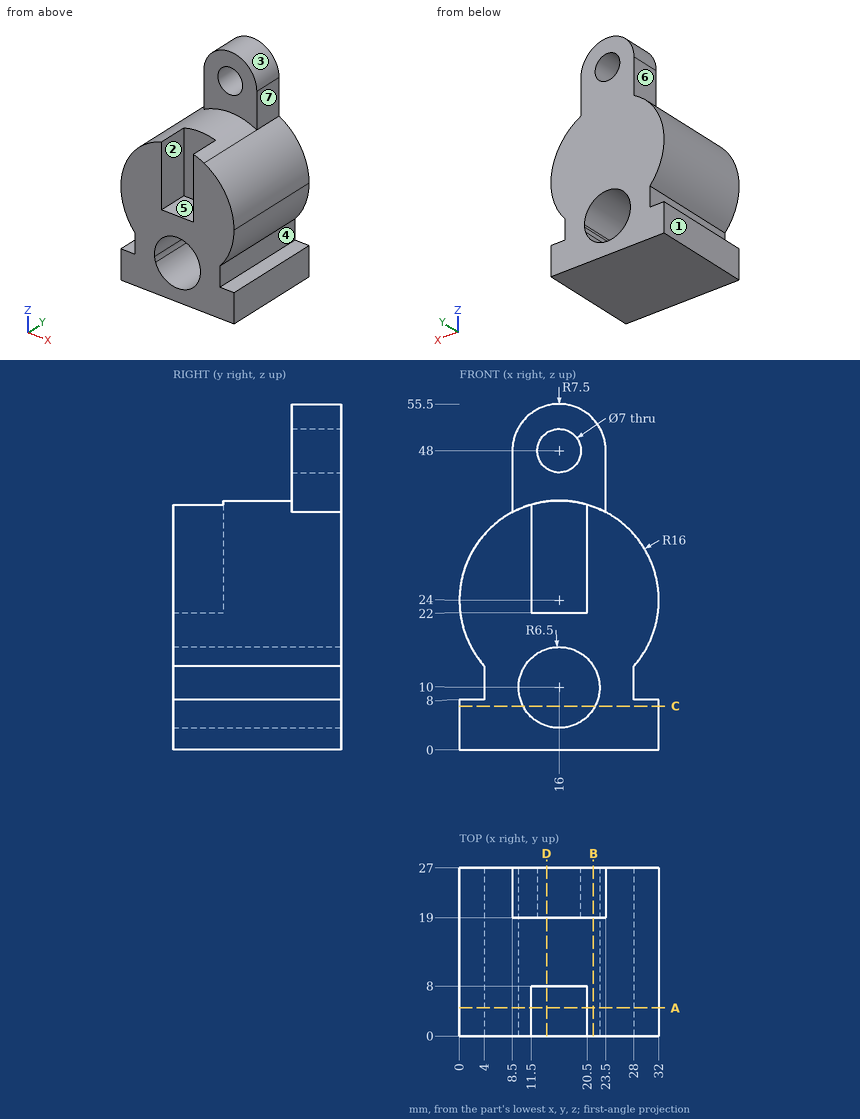
Drawing for the job (mm, zero at the part's lowest x, y, z). A direction names the side the tool comes from. Coordinates: 2 decimals unless noted, no trailing zeros. Order: outer loops, then holes, each group sorted by start corner. A loop starts at its lowest first (then second) coordinate and runs counter-clockwise, first axis right, second up. Notation, with made-up numbers: (-19, 23) - (5, 23) arc R21 ccw to (5, 56) - close; hole circle Ø9 at (-39, 68.5). An arc over 180 degrees is marked (long way). Use a Markdown table: item, result. Add a question column.
(1) Saw through at D-D (x = 14). Give the cut face in (y, z).
(2) Pull direction X, two halves, no side cores. Call the marked faces 1, 2 and 3: +X half, -X half, draft (parallel to the pull), parting line (faces both ways), or undercut.
(3) Which spindle directions (+Z, -Z, +X, -X, +Y, -Y) get a long thin tool onto all of the face, cutting with end or side? Do the marked faces 4, 5, 6 and 7. Say none if no direction does.
(4) Flat gauge pins, fed straight in: pin 1 (1.5 mm diameter, centred on x = 17.5, y = 10, fed in from +Z); pin 2 (3 mm diameter, centred on x = 7.5, z = 49, fed in from +Y); pin 3 (1.2 mm diameter, centred on x = 1.5, y = 15, fed in from +Z); pin 4 (1 mm diameter, centred on y = 16.5, z = 35.5, fed in from +X). Where does each tip first touch, or does it go through?
(5) Drill centre lines: line 1 along Z through (x, y) = (16, 22.75); line 2 along Y through (x, z) = (16.5, 37.5); line 3 along X through (y, z) = (25.5, 38.5). Where is each one in solid material? Low to high. Write a range as [from, to].
(6) Saw through at C-C (z = 7). Give the cut face in (x, y), then the cut area to 3 significant figures.
(7) Saw through at A-A (y = 4.5). Give the cut face in (x, z), then the cut area to 3 significant figures.
(8) Saw through at B-B (x = 21.5). Give the cut face in (y, z), then the cut area to 3 significant figures.
Solved:
| question | item | result |
|---|---|---|
| 1 | outline | (0, 0) - (27, 0) - (27, 3.82) - (0, 3.82) - close; (0, 16.18) - (27, 16.18) - (27, 45.13) - (19, 45.13) - (19, 39.87) - (8, 39.87) - (8, 22) - (0, 22) - close; (19, 50.87) - (27, 50.87) - (27, 55.23) - (19, 55.23) - close |
| 2 | face 1 | -X half |
| 2 | face 2 | undercut |
| 2 | face 3 | parting line |
| 3 | face 4 | +X, +Y, -Y |
| 3 | face 5 | +Z, -Y |
| 3 | face 6 | +Z, -X, +Y, -Y |
| 3 | face 7 | +Z, +X, +Y, -Y |
| 4 | pin 1 | stops at z = 39.98 |
| 4 | pin 2 | stops at y = 27 |
| 4 | pin 3 | stops at z = 31.92 |
| 4 | pin 4 | stops at x = 27.62 |
| 5 | line 1 | z = [0, 3.5], [16.5, 44.5], [51.5, 55.5] |
| 5 | line 2 | y = [8, 27] |
| 5 | line 3 | x = [8.5, 23.5] |
| 6 | outline | (0, 0) - (10.23, 0) - (10.23, 27) - (0, 27) - close; (21.77, 0) - (32, 0) - (32, 27) - (21.77, 27) - close |
| 6 | area | 553 mm² |
| 7 | outline | (0, 0) - (32, 0) - (32, 8) - (28, 8) - (28, 13.42) arc R16 ccw to (20.5, 39.35) - (20.5, 22) - (11.5, 22) - (11.5, 39.35) arc R16 ccw to (4, 13.42) - (4, 8) - (0, 8) - close; hole circle Ø13 at (16, 10) |
| 7 | area | 807 mm² |
| 8 | outline | (0, 0) - (27, 0) - (27, 6.54) - (0, 6.54) - close; (0, 13.46) - (27, 13.46) - (27, 53.1) - (19, 53.1) - (19, 39.02) - (0, 39.02) - close |
| 8 | area | 979 mm² |
